Autodesk Fusion 360 part; units mm, degrees
sketch "Sketch1" plane through (0, 0, 0) normal (1, 0, 0) x (0, 1, 0)
  line L0 (0, 25) -> (10, 25)
  line L1 (10, 25) -> (10, -25)
  line L2 (10, -25) -> (0, -25)
  arc A0 (0, 25) -> (0, -25) centre (0, 0) ccw
  line L3 (-60, 25) -> (-60, -25)
  dimension "d1" = 50
  dimension "d2" = 10
  dimension "d3" = 50
  dimension "d4" = 60
revolve "Revolve1" add sketch "Sketch1" angle 235 about axis through (0, -60, 25) along (0, 0, 1) makes body 1
sketch "Sketch2" plane through (0, 0, 25) normal (0, 0, 1) x (-1, 0, 0)
  line L0 (0, 0) -> (0, -10)
  arc A0 (0, -10) -> (-57.3406, 100.1504) centre (0, 60) ccw
  line L1 (-57.3406, 100.1504) -> (-49.1491, 94.4146)
  arc A1 (0, 0) -> (-49.1491, 94.4146) centre (0, 60) ccw
  line L2 (62.0908, 75) -> (120, 75)
  line L3 (120, 75) -> (120, 45)
  line L4 (120, 45) -> (62.0908, 45)
  line L5 (62.0908, 45) -> (62.0908, 75)
  line L6 (120, 75) -> (90, 75)
  line L7 (90, 75) -> (90, 45)
  line L8 (90, 45) -> (120, 45)
  line L9 (120, 45) -> (120, 75)
  line L10 (74.2462, 155.4594) -> (95.4594, 134.2462)
  line L11 (54.5114, 93.2982) -> (33.2982, 114.5114)
  line L12 (33.2982, 114.5114) -> (74.2462, 155.4594)
  line L13 (95.4594, 134.2462) -> (54.5114, 93.2982)
  line L14 (53.033, 134.2462) -> (74.2462, 113.033)
  line L15 (-15, 180) -> (15, 180)
  line L16 (15, 122.0908) -> (-15, 122.0908)
  line L17 (-15, 122.0908) -> (-15, 180)
  line L18 (15, 180) -> (15, 122.0908)
  line L19 (-15, 150) -> (15, 150)
  dimension "d6" = 30
  dimension "d7" = 120
  dimension "d8" = 15
  dimension "d9" = 30
  dimension "d10" = 30
  dimension "d12" = 90
extrude "Extrude1" add sketch "Sketch2" against normal blind 120 separate body contours L2 L3 L4 L6 L7 L8 L9 | L15 L17 L18 L19 | L10 L12 L13 L14 makes body 2 at (5, -150, -15) makes body 3 at (-60.1041, -127.1751, -15) makes body 4 at (-90, -65, -15)
extrude "Extrude2" add sketch "Sketch2" against normal blind 50 contours A0 L2 L4 L7 | A0 L17 L18 L19 | A0 L12 L13 L14 bodies 1 2 3 4
sketch "Sketch3" plane through (0, 0, -95) normal (0, 0, -1) x (1, 0, 0)
  line L0 (-53.033, 134.2462) -> (-74.2462, 155.4594)
  line L1 (-74.2462, 155.4594) -> (-95.4594, 134.2462)
  line L2 (-95.4594, 134.2462) -> (-74.2462, 113.033)
  line L3 (-74.2462, 113.033) -> (-53.033, 134.2462)
  line L4 (-15, 180) -> (-15, 128.374)
  line L5 (15, 180) -> (-15, 180)
  line L6 (15, 128.374) -> (15, 180)
  arc A0 (-15, 128.374) -> (-37.7411, 118.9543) centre (0, 60) ccw
  line L7 (-95.4594, 134.2462) -> (-58.9543, 97.7411)
  line L8 (-74.2462, 155.4594) -> (-95.4594, 134.2462)
  line L9 (-37.7411, 118.9543) -> (-74.2462, 155.4594)
  arc A1 (-58.9543, 97.7411) -> (-68.374, 75) centre (0, 60) ccw
  line L10 (-120, 75) -> (-68.374, 75)
  line L11 (-68.374, 45) -> (-120, 45)
  line L12 (-120, 45) -> (-120, 75)
  arc A2 (-68.374, 45) -> (0, -10) centre (0, 60) ccw
  line L13 (0, 0) -> (0, 25)
  line L14 (28.6703, 80.0752) -> (49.1491, 94.4146)
  arc A3 (57.3406, 100.1504) -> (15, 128.374) centre (0, 60) ccw
  line L15 (0, 0) -> (0, -10)
  line L16 (49.1491, 94.4146) -> (57.3406, 100.1504)
  arc A4 (28.6703, 80.0752) -> (0, 25) centre (0, 60) ccw
  circle A5 centre (0, 60) radius 35
  circle A6 centre (0, 60) radius 50
  line L17 (-15, 128.374) -> (15, 128.374)
  line L18 (15, 128.374) -> (15, 100.874)
  line L19 (15, 100.874) -> (-15, 100.874)
  line L20 (-15, 100.874) -> (-15, 128.374)
  line L21 (-39.5089, 78.2957) -> (-58.9543, 97.7411)
  line L22 (-58.9543, 97.7411) -> (-37.7411, 118.9543)
  line L23 (-18.2957, 99.5089) -> (-39.5089, 78.2957)
  line L24 (-37.7411, 118.9543) -> (-18.2957, 99.5089)
  line L25 (-40.874, 45) -> (-68.374, 45)
  line L26 (-68.374, 45) -> (-68.374, 75)
  line L27 (-40.874, 75) -> (-40.874, 45)
  line L28 (-68.374, 75) -> (-40.874, 75)
  dimension "d17" = 70
  dimension "d18" = 100
  dimension "d19" = 30
  dimension "d20" = 27.5
  dimension "d22" = 90
extrude "Extrude3" add sketch "Sketch3" against normal blind 20 contours L3 L7 L9 L22 | A6 L21 L22 L24 | L4 L5 L6 L17 | A6 L17 L18 L20 | A6 L21 L23 L24 | L13 L14 A4 A5 A6 L18 L19 L20 L21 L23 L24 L25 L27 L28 | L10 L11 L12 L26 | A6 L25 L26 L28 | A6 L18 L19 L20 | A6 L25 L27 L28 | L13 L14 A5 A6 bodies 1
Geometry check sheet. Reference: the model listing, model coordinates, mm. A direction names the side the tool comes from. Round coordinates to 2 decimals unless told otherwise and drop trailing zeros. Loops run counter-clockwise (first coordinate to the right, second up) from the corner with the lowest first, then second, coordinate; pieces in that order, holes last. Notation, with made-up numbers: M 2.25,-34.75 L 53.25,-34.75 A31 cw 53.25,0.25 Z; hole C 12.25,46 d5. An arc over 180 degrees is marked long. Return JSON: item names as keys, results as strings. Group by question number.
(1) Set-up check for faces 1 (the face through (-90, -60, -50)), 2 (the face through (45.99, -92.203, 0.35)), 3 (the face through (-26.628, -124.738, -0.35)): record each of +Z, -Z, +X, -X, +Y, -Y from which the full face is reachable in a straight line by a thin tool's end or side.
(2) Mould release check, pull along Y, two halves, no side actions. Record for faces 4 (the face through (-64.605, -86.948, -0.35)), 5 (the face through (-44.39, -5.875, -0.35)), 6 (the face through (-59.687, -140.9, -34.16)): pulls with the +Y half, pulls with the -Y half, needs draft (parallel to the pull), parting line crosses it, or undercut.
(3) Section check B-B, the plane y = -60. Enter the section's corners in (x, z), and give its area (3 significant figures).
(4) Go/stop test with flat-tipped pins: pin 1 (17.5 mm diameter, centred on y = 1, z = -7.5, fed in from +X); pin 2 (9 mm diameter, centred on x = 0, z = -52, fed in from +Y); pin 3 (21.5 mm diameter, centred on y = -153, z = -9, fed in from +X). Record where each tip stops, or that it passes through.
(5) Section check D-D, the plane z = -13. Enter the section's corners in (x, y).
(6) Scan lines: line 1 along Z through (x, y) = (-57, -96); line 2 along Y through (x, z) = (-96, -61.5); line 3 along Y through (x, z) = (-1, -64.5). Record each from-to range of solid material in increasing order. Write a range as [from, to].
(7) Section check C-C, the plane x = 21. Give the number of separate pieces and of enclosed holes in the cut face, and give its area (3 significant figures).
(8) Section check A-A, the plane z = -54. Enter the section's corners in (x, y), and give its area (3 significant figures).
Data:
{
 "1": {"face 1": "+X, +Y", "face 2": "+Z, +X, +Y", "face 3": "+Z, -Z, -Y"},
 "2": {"face 4": "undercut", "face 5": "pulls with the +Y half", "face 6": "pulls with the -Y half"},
 "3": {"outline": "M -120,-95 L -35,-95 L -35,-75 L -90,-75 L -90,-25 L -60,-25 A25 ccw -60,25 L -120,25 Z; M 35,-95 L 50,-95 L 50,-75 L 35,-75 Z", "area": "7,480 mm²"},
 "4": {"pin 1": "x = 0", "pin 2": "y = -150", "pin 3": "x = 15"},
 "5": {"outline": "M -120,-75 L -68.37,-75 A70 ccw -58.95,-97.74 L -95.46,-134.25 L -74.25,-155.46 L -37.74,-118.95 A70 ccw -15,-128.37 L -15,-180 L 15,-180 L 15,-128.37 A70 ccw 57.34,-100.15 L 31.66,-82.17 A38.65 cw long 0,-21.35 L 0,10 A70 ccw -68.37,-45 L -120,-45 Z"},
 "6": {"line 1": "[-95, -75], [-25, 25]", "line 2": "[-75, -45]", "line 3": "[-180, -150]"},
 "7": {"separate pieces": "3", "enclosed holes": "0", "area": "2,320 mm²"},
 "8": {"outline": "M -120,-75 L -90,-75 L -90,-45 L -120,-45 Z; M -95.46,-134.25 L -74.25,-155.46 L -53.03,-134.25 L -74.25,-113.03 Z; M -15,-180 L 15,-180 L 15,-150 L -15,-150 Z", "area": "2,700 mm²"}
}
